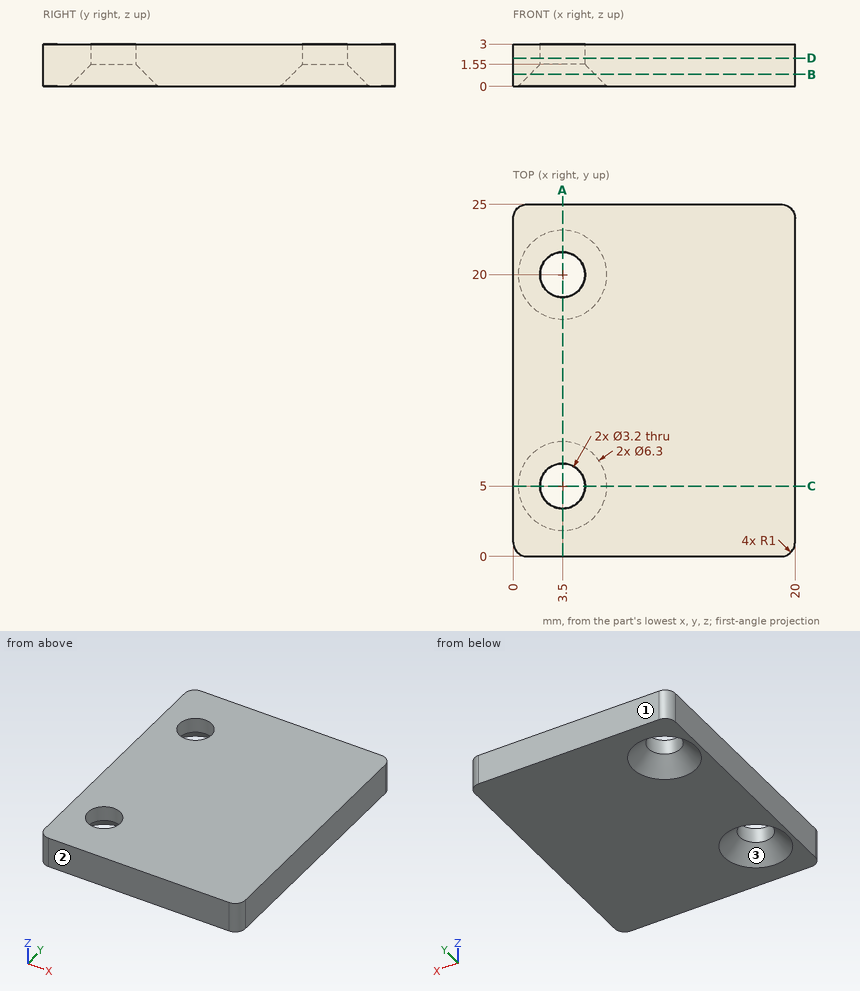
Design review of the part shown in the three views and the two pictorial views. Dimensions are in mm from the part's minimum x, y and z. Give positions to 0.01 mm unless a question says otherwise; leave off trailing zeros. Loops run counter-clockwise (first coordinate to the right, second up) from the corner with the lowest first, then second, coordinate; pieces in that order, holes last. Notation, with made-up numbers: (85, -33.75) -> (128, -33.75) arc R16 cw to (128, -24.75) -> close; hole circle Ø5 at (23, 69.25). An arc over 180 degrees is marked (long way). Put each result on its own line as item: value. Start each with the question number.
1. Wall thickness on probe 1 along Y at (x, z) = (3.5, 2); probe 2 along X at (y, z) = (5, 2.4); probe 3 along Y at (x, z) = (3.25, 0.65): over which ranges is each line inside the solid? List them lowest first.
2. We need section A-A on x = 3.5. State the section outline as (y, z) points.
3. We need section D-D on z = 2. State the section outline as (x, y) points.
4. Clearance check with a flat-ended pin moving along its axis: P1, Ø5, axis at x = 3.5, y = 5, coming from the -Z side. State where the tip first meets the part, or that it passes through.
5. We need section C-C on y = 5. State the section outline as (x, z) points.
6. We need section B-B on z = 0.85. State the section outline as (x, y) points.
7. Mouldability with a two-part tool opening along Y and no side actions: class the marked faces 1, 2 and 3 as released by +Y, released by -Y, zero draft, split by the parting line, or undercut.
Determined:
1. probe 1: 0 to 3.4, 6.6 to 18.4, 21.6 to 25
1. probe 2: 0 to 1.9, 5.1 to 20
1. probe 3: 0 to 2.51, 7.49 to 17.51, 22.49 to 25
2. outline: (0, 0) -> (1.85, 0) -> (3.4, 1.55) -> (3.4, 3) -> (0, 3) -> close; (6.6, 1.55) -> (8.15, 0) -> (16.85, 0) -> (18.4, 1.55) -> (18.4, 3) -> (6.6, 3) -> close; (21.6, 1.55) -> (23.15, 0) -> (25, 0) -> (25, 3) -> (21.6, 3) -> close
3. outline: (0, 1) arc R1 ccw to (1, 0) -> (19, 0) arc R1 ccw to (20, 1) -> (20, 24) arc R1 ccw to (19, 25) -> (1, 25) arc R1 ccw to (0, 24) -> close; hole circle Ø3.2 at (3.5, 5); hole circle Ø3.2 at (3.5, 20)
4. P1: z = 0.65
5. outline: (0, 0) -> (0.35, 0) -> (1.9, 1.55) -> (1.9, 3) -> (0, 3) -> close; (5.1, 1.55) -> (6.65, 0) -> (20, 0) -> (20, 3) -> (5.1, 3) -> close
6. outline: (0, 1) arc R1 ccw to (1, 0) -> (19, 0) arc R1 ccw to (20, 1) -> (20, 24) arc R1 ccw to (19, 25) -> (1, 25) arc R1 ccw to (0, 24) -> close; hole circle Ø4.6 at (3.5, 5); hole circle Ø4.6 at (3.5, 20)
7. face 1: released by +Y
7. face 2: released by -Y
7. face 3: undercut
